The model under review builds one solid part; all positions refer to its coordinate system, in mm. A direction names the side the tool comes from. Round coordinates to 2 decimals unless told otherwise and drop trailing zeros. Order: outer loops, then holes, each group sorted by start corner. A loop starts at its lowest first (then second) coordinate and runs counter-clockwise, first axis right, second up. Notation, with made-up numbers: M -0.75,-33.75 L 41.25,-33.75 A33 ccw 41.25,-3.75 Z; hole C 46,-39 d4. An arc over 180 degrees is marked long. Answer as a JSON object with one key per item and string values. Group by question number.
1) Insertion check: pin 1 Ø2.5 at (y, z) = (0, 0) entering from -X. The pin has a flat end and moves straight along its axis. Give the tip position at first contact, or say it passes through.
2) To check wall thickness, follow line 1 (Z direction, x = 2.75, y = 0); line 2 (X direction, y = -0.75, z = -2.6); line 3 (Y direction, x = 5.75, z = -0.8). State the ranges of each line that lie inside material, in increasing order.
3) Consider section D-D, the plane z = 2.55. Write out the cut boundary in (x, y).
4) Consider section C-C, the plane z = -2.3. Write out the cut boundary in (x, y), then the cut area to 3 significant figures.
5) The part is to be moulded in two halves that separate along Y. For faces 3 (the conical face through (12.605, -0.275, -0.061)), 4 (the flat face through (0, 1.5, 1.4)), 5 (the cylindrical face through (19, 2, 0)), 6 (the cylindrical face through (5.983, 1.438, 0.748)), say which applies: +Y half, -Y half, draft (parallel to the pull), parting line (faces both ways), or undercut.
6) For faces 1 (the flat face through (23, 0, 0)), 2 (the flat face through (15, 1, 2)), list the 3-axis set-ups (+Z, -Z, +X, -X, +Y, -Y) from which the entire face can be reached by the end or side of a thin tool; tool diameter is ignored.
7) Consider section B-B, the plane x = 14.5. Write out the cut boundary in (y, z).
8) Consider section A-A, the plane x = 6.75. Write out the cut boundary in (y, z), then the cut area to 3 significant figures.
Autodesk Inventor part; units mm, degrees
ref_plane "YZ Plane" through (0, 0, 0) normal (1, 0, 0) x (0, 1, 0)
ref_plane "XZ Plane" through (0, 0, 0) normal (0, 1, 0) x (-1, 0, 0)
ref_plane "XY Plane" through (0, 0, 0) normal (0, 0, 1) x (1, 0, 0)
sketch "スケッチ1" plane through (0, 0, 0) normal (1, 0, 0) x (0, 1, 0)
  line L0 (1.7321, -3) -> (-1.7321, -3)
  line L1 (-1.7321, -3) -> (-3.4641, 0)
  line L2 (-3.4641, 0) -> (-1.7321, 3)
  line L3 (-1.7321, 3) -> (1.7321, 3)
  line L4 (1.7321, 3) -> (3.4641, 0)
  line L5 (3.4641, 0) -> (1.7321, -3)
  point P0 (0, 0)
  point P1 (0, 0)
  dimension "d0" = 6
extrude "押し出し1" add sketch "スケッチ1" along normal blind 15
sketch "スケッチ2" plane through (15, 0, 0) normal (1, 0, 0) x (0, 0, -1)
  circle A0 centre (0, 0) radius 2
  dimension "d3" = 4
extrude "押し出し2" add sketch "スケッチ2" along normal blind 8
thread "ねじ1"
sketch "スケッチ3" plane through (0, 0, 0) normal (-1, 0, 0) x (0, 0, 1)
  point P0 (0, 0)
  point P1 (0, 0)
hole "穴1" at (0, 0, 0) direction (1, 0, 0) diameter 3.242 depth 11.8 tip angle 118
properties part number "Spacer_M3_L15" material "鋼、合金"
Results list:
{
 "1": {"pin 1": "x = 12.02"},
 "2": {"line 1": "-3 to -1.62, 1.62 to 3", "line 2": "0 to 15", "line 3": "-3 to -1.41, 1.41 to 3"},
 "3": {"outline": "M 0,-1.99 L 15,-1.99 L 15,1.99 L 0,1.99 Z"},
 "4": {"outline": "M 0,-2.14 L 15,-2.14 L 15,2.14 L 0,2.14 Z", "area": "64.1 mm^2"},
 "5": {"face 3": "undercut", "face 4": "draft", "face 5": "parting line", "face 6": "undercut"},
 "6": {"face 1": "+Z, -Z, +X, +Y, -Y", "face 2": "+X"},
 "7": {"outline": "M -3.46,0 L -1.73,-3 L 1.73,-3 L 3.46,0 L 1.73,3 L -1.73,3 Z"},
 "8": {"outline": "M -3.46,0 L -1.73,-3 L 1.73,-3 L 3.46,0 L 1.73,3 L -1.73,3 Z; hole C 0,0 d3.24", "area": "22.9 mm^2"}
}
